Verification items for the finished model (mm, model axes). A direction names the side the tool comes from. Round coordinates to 2 decimals unless told otherwise and drop trailing zeros. Order: outer loops, then holes, each group sorted by start corner. A loop starts at its lowest first (then second) coordinate and runs counter-clockwise, first axis right, second up. Notation, with made-up numbers: (-12, 47) -> (39, 47) arc R29 ccw to (39, 78) -> close; hole circle Ø7 at (22.5, 42.5). An arc over 180 degrees is marked (long way). Answer in a Markdown table with one row per item. Add a question column.
Autodesk Inventor part; units mm, degrees
ref_plane "YZ Plane" through (0, 0, 0) normal (1, 0, 0) x (0, 1, 0)
ref_plane "XZ Plane" through (0, 0, 0) normal (0, 1, 0) x (-1, 0, 0)
ref_plane "XY Plane" through (0, 0, 0) normal (0, 0, 1) x (1, 0, 0)
sketch "Sketch1" plane through (0, 0, 0) normal (0, 1, 0) x (-1, 0, 0)
  line L0 (0, 0) -> (25.4, 0)
  line L1 (25.4, 0) -> (25.4, -88.9)
  line L2 (25.4, -88.9) -> (0, -88.9)
  line L3 (0, -88.9) -> (0, 0)
  dimension "d0" = 88.9
  dimension "d1" = 25.4
extrude "Extrusion1" add sketch "Sketch1" along normal blind 50.8
shell "Shell1" thickness 2.54 removed faces 2 at (-16.9333, 33.8667, 0) at (-8.4667, 16.9333, -88.9)
sketch "Sketch2" plane through (0, 50.8, 0) normal (0, 1, 0) x (1, 0, 0)
  line L0 (-2.54, 0) -> (-22.86, 0) construction
  line L1 (-12.7, 0) -> (-12.7, 62.6675) construction
  circle A0 centre (-12.7, 0) radius 2.0701
  circle A1 centre (-12.7, 12.7) radius 2.0701
  circle A2 centre (-12.7, 25.4) radius 2.0701
  circle A3 centre (-12.7, 38.1) radius 2.0701
  circle A4 centre (-12.7, 50.8) radius 2.0701
  point P0 (0, 0)
  dimension "d5" = 4.1402
  dimension "d8" = 12.7
extrude "Extrusion2" cut sketch "Sketch2" against normal through all contours A1 | A2 | A3 | A4
1) Thickness scan on L1, parallel to Z at x = -12.7, y = 0.6; L2, parallel to X at y = 6, z = -7; L3, parallel to Y at x = -14.5, z = -58.5. Record the ranges inside material, lowest first. Write a range as [from, to].
2) Depth check by flat-ended pin: P1, Ø2.5, axis at x = -12.7, z = -12.7, coming from the +Y side. Enter the tip coordinate at first touch or a pass-through.
3) Cross-section at A-A, the plane y = 27.5. Record the boundary of the cut face in (x, z).
4) Cross-section at C-C, the plane x = -15.75. Record the boundary of the cut face in (y, z), and give its area (3 significant figures).
5) Draft check along Y on faces 1 (the face through (-13, 48.26, -44)), 2 (the face through (-13, 0, -44)), 3 (the face through (-14.34, 1.29, -24.14)). Enter one of: +Y half, -Y half, draft (parallel to the pull), parting line (faces both ways), or undercut.
6) Cross-section at B-B, the plane z = -60.5. Record the boundary of the cut face in (x, y), and give its area (3 significant figures).
7) Tool access check on faces 4 (the face through (-13.15, 1.29, -36.08)), 5 (the face through (-13, 2.54, -44)). Record the directions out of +Z, -Z, +X, -X, +Y, -Y that give a thin tool (end or side, any length) a straight path to the whole face; none if there is none.
8) Cross-section at D-D, the plane z = -12.7. Record the boundary of the cut face in (x, y).
Results below:
| question | item | result |
|---|---|---|
| 1 | L1 | [-88.9, -52.87], [-48.73, -40.17], [-36.03, -27.47], [-23.33, -14.77], [-10.63, 0] |
| 1 | L2 | [-25.4, -22.86], [-2.54, 0] |
| 1 | L3 | [0, 2.54], [48.26, 50.8] |
| 2 | P1 | through |
| 3 | outline | (-25.4, -88.9) -> (-22.86, -88.9) -> (-22.86, 0) -> (-25.4, 0) -> close; (-2.54, -88.9) -> (0, -88.9) -> (0, 0) -> (-2.54, 0) -> close |
| 4 | outline | (0, -88.9) -> (2.54, -88.9) -> (2.54, 0) -> (0, 0) -> close; (48.26, -88.9) -> (50.8, -88.9) -> (50.8, 0) -> (48.26, 0) -> close |
| 4 | area | 452 mm² |
| 5 | face 1 | undercut |
| 5 | face 2 | -Y half |
| 5 | face 3 | draft |
| 6 | outline | (-25.4, 0) -> (0, 0) -> (0, 50.8) -> (-25.4, 50.8) -> close; hole (-22.86, 2.54) -> (-2.54, 2.54) -> (-2.54, 48.26) -> (-22.86, 48.26) -> close |
| 6 | area | 361 mm² |
| 7 | face 4 | +Y, -Y |
| 7 | face 5 | +Z, -Z |
| 8 | outline | (-25.4, 0) -> (-14.77, 0) -> (-14.77, 2.54) -> (-22.86, 2.54) -> (-22.86, 48.26) -> (-14.77, 48.26) -> (-14.77, 50.8) -> (-25.4, 50.8) -> close; (-10.63, 0) -> (0, 0) -> (0, 50.8) -> (-10.63, 50.8) -> (-10.63, 48.26) -> (-2.54, 48.26) -> (-2.54, 2.54) -> (-10.63, 2.54) -> close |
